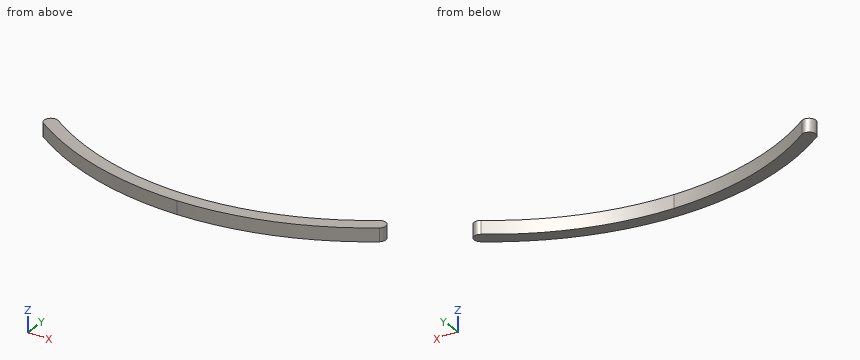
Autodesk Inventor part; units mm, degrees
ref_plane "YZ Plane" through (0, 0, 0) normal (1, 0, 0) x (0, 1, 0)
ref_plane "XZ Plane" through (0, 0, 0) normal (0, 1, 0) x (-1, 0, 0)
ref_plane "XY Plane" through (0, 0, 0) normal (0, 0, 1) x (1, 0, 0)
sketch "Sketch1" plane through (0, 0, 0) normal (0, 0, 1) x (1, 0, 0)
  arc A0 (0, -2125) -> (1212.8796, -1744.8633) centre (0, 0) ccw
  arc A1 (0, -2225) -> (1269.9563, -1826.9745) centre (0, 0) ccw
  line L0 (0, -2125) -> (0, -1744.8633)
  arc A2 (1269.9563, -1826.9745) -> (1212.8796, -1744.8633) centre (1241.418, -1785.9189) ccw
  line L1 (0, -2225) -> (0, -2125)
  arc A3 (-1212.8796, -1744.8633) -> (0, -2125) centre (0, 0) ccw
  arc A4 (-1269.9563, -1826.9745) -> (0, -2225) centre (0, 0) ccw
  arc A5 (-1212.8796, -1744.8633) -> (-1269.9563, -1826.9745) centre (-1241.418, -1785.9189) ccw
  dimension "d0" = 4250
  dimension "d1" = 4450
extrude "Extrusion1" add sketch "Sketch1" along normal blind 100
properties part number "Saddle"
CAD build for the part. Positions are in the model's coordinates, mm. Coordinates: 2 decimals unless noted, no trailing zeros. Write each loop counter-clockwise with the first axis right and the second up, starting at its lowest first coordinate (ties: lowest second). Pieces come first, ordered by that corner, then holes.
(1) Cut at C-C, the plane y = -1857.5. List the corners of the cut face in (x, z).
(2) Flat gauge pins, fed straight in: pin 1 (12 mm diameter, centred on y = -2038, z = 13, fed in from -X); pin 2 (3 mm diameter, centred on y = -2052, z = 80, fed in from -X); pin 3 (8 mm diameter, centred on x = 947, z = 90, fed in from +Y). Where does each tip first touch, or does it go through?
(3) Cut at B-B, the plane z = 32. List the corners of the cut face in (x, y), and give its area (3 significant figures).
(4) Drill centre lines: probe 1 along X at (y, z) = (-1832, 51); probe 2 along X at (y, z) = (-1859.5, 58.5); probe 3 along Y at (x, z) = (1000.5, 9). Where is each one in solid material? Low to high.
(5) Cut at D-D, the plane x = -61. List the corners of the cut face in (y, z), and give its area (3 significant figures).
(6) Cut at A-A, the plane y = -2046. List the corners of the cut face in (x, z), and give its area (3 significant figures).
Geometry says:
1. outline: (-1224.87, 0) - (-1032.14, 0) - (-1032.14, 100) - (-1224.87, 100) - close; (1032.14, 0) - (1224.87, 0) - (1224.87, 100) - (1032.14, 100) - close
2. pin 1: stops at x = -906.42
2. pin 2: stops at x = -863.76
2. pin 3: stops at y = -1900.32
3. outline: (-1269.96, -1826.97) arc R2225 ccw to (0, -2225) arc R2225 ccw to (1269.96, -1826.97) arc R50 ccw to (1212.88, -1744.86) arc R2125 cw to (0, -2125) arc R2125 cw to (-1212.88, -1744.86) arc R50 ccw to start
3. area: 272,000 mm2
4. probe 1: x = -1262.7 to -1076.75, 1076.75 to 1262.7
4. probe 2: x = -1221.84 to -1028.54, 1028.54 to 1221.84
4. probe 3: y = -1987.37 to -1874.73
5. outline: (-2224.16, 0) - (-2124.12, 0) - (-2124.12, 100) - (-2224.16, 100) - close
5. area: 10,000 mm2
6. outline: (-874.36, 0) - (-574.03, 0) - (-574.03, 100) - (-874.36, 100) - close; (574.03, 0) - (874.36, 0) - (874.36, 100) - (574.03, 100) - close
6. area: 60,100 mm2
